The drawing under review shows one solid part. Ordinate dimensions are in mm from its lowest x, y, z. A direction names the side the tool comes from. Round coordinates to 2 decimals unless told otherwise and drop trailing zeros. Write each loop counter-clockwise with the first axis right and the second up, starting at its lowest first coordinate (ties: lowest second). Pieces come first, ordered by that corner, then holes. Notation, with made-up numbers: (28, 7) -> (73, 7) arc R33 ccw to (73, 37) -> close; hole circle Ø2 at (76.25, 59). An arc over 180 degrees is marked (long way). Answer in a Markdown table with one row per item.
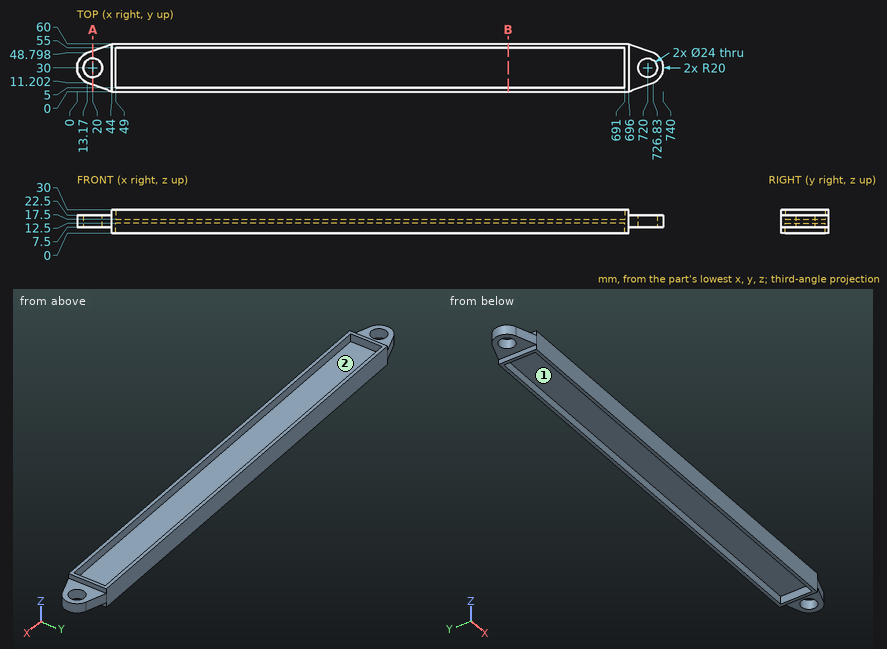
1) Consider section B-B on x = 544. State the section outline as (y, z) points, then the cut area to 3 significant figures.
Solved:
| item | result |
|---|---|
| outline | (0, 0) -> (5, 0) -> (5, 12.5) -> (55, 12.5) -> (55, 0) -> (60, 0) -> (60, 30) -> (55, 30) -> (55, 17.5) -> (5, 17.5) -> (5, 30) -> (0, 30) -> close |
| area | 550 mm² |
2) Clearance check with flat-ended pins moving along their axes: pin 1 Ø4 at (y, z) = (40, 9) entering from +X; pin 2 Ø10 at (y, z) = (20.5, 26.5) entering from -X (1 decimal); pin 3 Ø3 at (x, y) = (428, 45) entering from +Z; pin 4 Ø21.5 at (x, y) = (720, 30) entering from +Z. State where each tip first meets the part, or that it passes through.
Solved:
| item | result |
|---|---|
| pin 1 | x = 738.33 |
| pin 2 | x = 1.1 |
| pin 3 | z = 17.5 |
| pin 4 | through |
3) For line 1 (X direction, y = 25, z = 25.25); line 2 (Y direction, x = 649, z = 23.75); line 3 (X direction, y = 21, z = 9) (1 decimal), list the stretches that pass through material, from the lowest coordinate up. Write a range as [from, to].
Solved:
| item | result |
|---|---|
| line 1 | [44, 49], [691, 696] |
| line 2 | [0, 5], [55, 60] |
| line 3 | [2.1, 12.1], [27.9, 49], [691, 712.1], [727.9, 737.9] |
4) Consider section A-A on x = 20. State the section outline as (y, z) points.
Solved:
| item | result |
|---|---|
| outline | (8.72, 7.5) -> (18, 7.5) -> (18, 22.5) -> (8.72, 22.5) -> close; (42, 7.5) -> (51.28, 7.5) -> (51.28, 22.5) -> (42, 22.5) -> close |
5) For the marked faces 1 and 2, list the 3-axis set-ups (+Z, -Z, +X, -X, +Y, -Y) from which the entire face can be reached by the end or side of a thin tool; tool diameter is ignored.
Solved:
| item | result |
|---|---|
| face 1 | -Z |
| face 2 | +Z |
